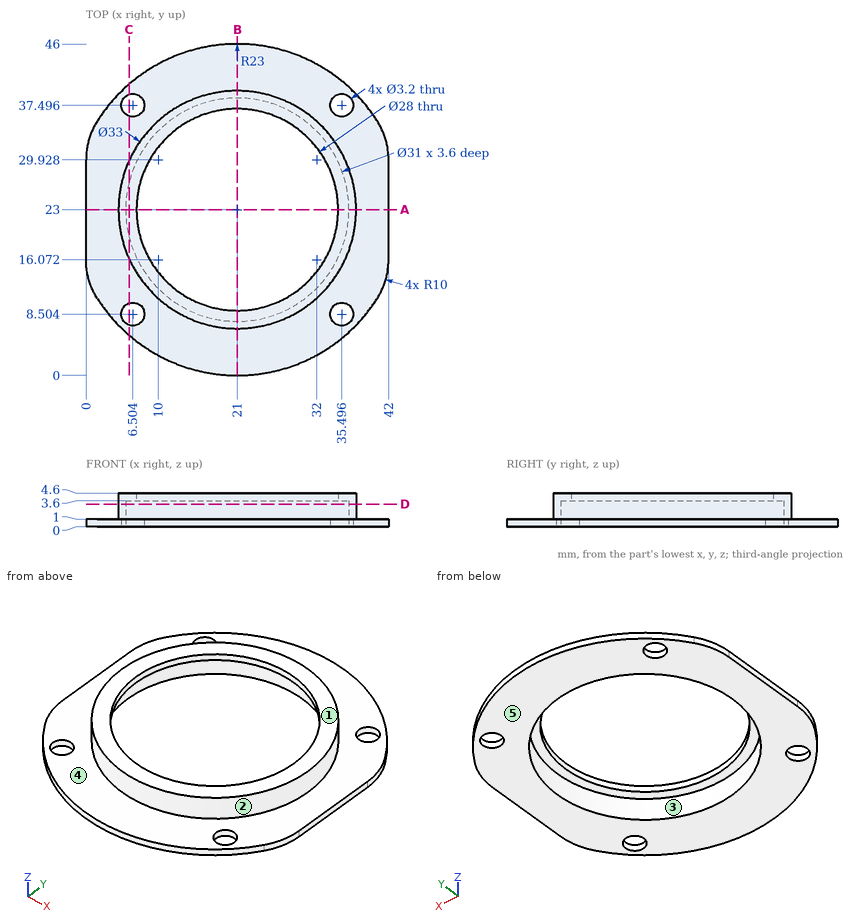
Job drawing, mm, ordinate dimensions from the low corner. One solid piece. A direction names the side the tool comes from. Coordinates: 2 decimals unless noted, no trailing zeros. Write each loop counter-clockwise with the first axis right and the second up, starting at its lowest first coordinate (ties: lowest second). Pieces come first, ordered by that corner, then holes. Notation, with made-up numbers: (1, 87.25) - (22, 87.25) arc R12 ccw to (22, 91.25) - close; hole circle Ø1 at (84, 30). An arc over 180 degrees is marked (long way). Use a Markdown table: item, result. Add a question column.
Item 1: Drill centre lines: L1, parallel to Y at x = 21, z = 4; L2, parallel to Z at x = 28.5, y = 11; L3, parallel to X at y = 33.5, z = 0.55. Where is each one in solid material? Low to high. Write a range as from..to.
Item 2: Band-saw the part on D-D, the plane z = 3.1. Give the cut face in (x, y).
Item 3: Band-saw the part on A-A, the plane y = 23. Give the cut face in (x, z), and give its area (3 significant figures).
Item 4: Band-saw the part on C-C, the plane x = 6. Give the cut face in (y, z) (1 decimal).
Item 5: 3-axis set-ups, long thin cutter, end or side, ignore diameter. For the marked faces 4 and 5: which of +Z, -Z, +X, -X, +Y, -Y reach the whole face in a straight line?
Item 6: Flat gauge pins, fed straight in: pin 1 (1.9 mm diameter, centred on x = 6.5, y = 8.5, fed in from -Z); pin 2 (1.5 mm diameter, centred on x = 31.5, z = 2.5, fed in from +Y); pin 3 (1.5 mm diameter, centred on x = 22, z = 3.5, fed in from -Y). Where does each tip first touch, or does it go through?
Item 7: Band-saw the part on B-B, the plane x = 21. Give the cut face in (y, z), and give its area (3 significant figures).
Item 8: Mould opens along X. For the marked faces 1, 2 and 3 say: pulls with the +X half, pulls with the -X half, needs draft (parallel to the pull), parting line crosses it, or undercut.
Numbers:
| question | item | result |
|---|---|---|
| 1 | L1 | 6.5..9, 37..39.5 |
| 1 | L2 | 3.6..4.6 |
| 1 | L3 | 0.66..9.6, 32.4..41.34 |
| 2 | outline | circle Ø33 at (21, 23); hole circle Ø31 at (21, 23) |
| 3 | outline | (0, 0) - (5.5, 0) - (5.5, 3.6) - (7, 3.6) - (7, 4.6) - (4.5, 4.6) - (4.5, 1) - (0, 1) - close; (35, 3.6) - (36.5, 3.6) - (36.5, 0) - (42, 0) - (42, 1) - (37.5, 1) - (37.5, 4.6) - (35, 4.6) - close |
| 3 | area | 21.2 mm2 |
| 4 | outline | (5.6, 0) - (7, 0) - (7, 1) - (5.6, 1) - close; (10, 0) - (19.1, 0) - (19.1, 3.6) - (26.9, 3.6) - (26.9, 0) - (36, 0) - (36, 1) - (29.9, 1) - (29.9, 4.6) - (16.1, 4.6) - (16.1, 1) - (10, 1) - close; (39, 0) - (40.4, 0) - (40.4, 1) - (39, 1) - close |
| 5 | face 4 | +Z |
| 5 | face 5 | -Z, +X, -X, +Y, -Y |
| 6 | pin 1 | through |
| 6 | pin 2 | y = 36.31 |
| 6 | pin 3 | y = 6.5 |
| 7 | outline | (0, 0) - (7.5, 0) - (7.5, 3.6) - (9, 3.6) - (9, 4.6) - (6.5, 4.6) - (6.5, 1) - (0, 1) - close; (37, 3.6) - (38.5, 3.6) - (38.5, 0) - (46, 0) - (46, 1) - (39.5, 1) - (39.5, 4.6) - (37, 4.6) - close |
| 7 | area | 25.2 mm2 |
| 8 | face 1 | needs draft |
| 8 | face 2 | parting line crosses it |
| 8 | face 3 | undercut |
